from build123d import *

# Parameters (mm, degrees)
SKETCH1_W           = 38.1
SKETCH1_H           = 38.1
SKETCH1_R           = 1.0795
BOSS_EXTRUDE1_DEPTH = 1.5875
SKETCH3_W           = 10.16
SKETCH3_H           = 5.08
BOSS_EXTRUDE2_DEPTH = 8.89
SKETCH4_R           = 8.255
BOSS_EXTRUDE3_DEPTH = 16.637


with BuildPart() as part:
    # Sketch1 → Boss-Extrude1 (new body)
    with BuildSketch(Plane(origin=(0, 0, 0), x_dir=(0, 0, -1), z_dir=(1, 0, 0))):
        Rectangle(SKETCH1_W, SKETCH1_H)
        with Locations((13.97, -13.97)):
            Circle(SKETCH1_R, mode=Mode.SUBTRACT)
        with Locations((-13.97, -13.97)):
            Circle(SKETCH1_R, mode=Mode.SUBTRACT)
        with Locations((-13.97, 13.97)):
            Circle(SKETCH1_R, mode=Mode.SUBTRACT)
        with Locations((13.97, 13.97)):
            Circle(SKETCH1_R, mode=Mode.SUBTRACT)
    extrude(amount=BOSS_EXTRUDE1_DEPTH)

    # Sketch3 → Boss-Extrude2 (add)
    with BuildSketch(Plane.ZY):
        with Locations((-6.35, -12.7)):
            Rectangle(SKETCH3_W, SKETCH3_H)
    extrude(amount=BOSS_EXTRUDE2_DEPTH)

    # Sketch4 → Boss-Extrude3 (add)
    with BuildSketch(Plane(origin=(1.5875, 0, 0), x_dir=(0, 0, -1), z_dir=(1, 0, 0))):
        Circle(SKETCH4_R)
    extrude(amount=BOSS_EXTRUDE3_DEPTH)


solid = part.part
The listing builds one solid part. Answer for the finished solid, in the listing's coordinates (mm). A direction names the side the tool comes from. Coordinates: 2 decimals unless noted, no trailing zeros. Loops run counter-clockwise (first coordinate to the right, second up) from the corner with the lowest first, then second, coordinate; pieces in that order, holes last. Notation, with made-up numbers: (-19.75, 69) -> (33.25, 69) arc R18 ccw to (33.25, 94) -> close; hole circle Ø2 at (81, 71). An arc over 180 degrees is marked (long way). Answer in a Markdown table with one row per item. Add a question column.
1. For faces 1 (the flat face through (-4, -15.24, -6)), 2 (the flat face through (-4, -13, -1.27)), 3 (the flat face through (-4, -10.16, -6)), 4 (the cylindrical face through (9.79, 2.48, -7.874)), determine the directions among +Z, -Z, +X, -X, +Y, -Y from which every point of the face is accessible in a straight line to the end or side of a thin tool.
2. The part is cut by section D-D, the plane x = -5.75. Write down the section's boundary in (y, z).
3. Determine the mould class of faces 5 (the flat face through (-4, -13, -11.43)), 6 (the flat face through (1, -19.05, 0)), 7 (the cylindrical face through (0.78, -14.38, -14.97)) for opening direction Z: +Z half, -Z half, draft (parallel to the pull), parting line (faces both ways), or undercut.
4. The part is cut by section B-B, the plane z = -13.97. Write down the section's boundary in (x, y), then the cut area to 3 significant figures.
5. Consider line 1 (Y direction, x = 1, z = -13.97); line 2 (X direction, y = -12.5, z = 12); line 3 (X direction, y = 1, z = 3.5). Determine where each line is inside the solid, lowest interval first. Write a range as [from, to].
6. Flat-ended cylindrical pins translate along their axes: P1, Ø3, axis at y = 9.5, z = -3.5, coming from the -X side; P2, Ø4.5, axis at x = -5.5, z = -5, coming from the +Y side; P3, Ø2.5, axis at x = -4, z = -6, coming from the -Y side. Find the tip coordinate at first contact, or state that the pin passes through.
7. The part is cut by section A-A, the plane y = -13.97. Write down the section's boundary in (x, z).
Answer below:
| question | item | result |
|---|---|---|
| 1 | face 1 | +Z, -Z, -X, -Y |
| 1 | face 2 | +Z, -X, +Y, -Y |
| 1 | face 3 | +Z, -Z, -X, +Y |
| 1 | face 4 | +X |
| 2 | outline | (-15.24, -11.43) -> (-10.16, -11.43) -> (-10.16, -1.27) -> (-15.24, -1.27) -> close |
| 3 | face 5 | -Z half |
| 3 | face 6 | draft |
| 3 | face 7 | undercut |
| 4 | outline | (0, -19.05) -> (1.59, -19.05) -> (1.59, -15.05) -> (0, -15.05) -> close; (0, -12.89) -> (1.59, -12.89) -> (1.59, 12.89) -> (0, 12.89) -> close; (0, 15.05) -> (1.59, 15.05) -> (1.59, 19.05) -> (0, 19.05) -> close |
| 4 | area | 53.6 mm2 |
| 5 | line 1 | [-19.05, -15.05], [-12.89, 12.89], [15.05, 19.05] |
| 5 | line 2 | [0, 1.59] |
| 5 | line 3 | [0, 18.22] |
| 6 | P1 | x = 0 |
| 6 | P2 | y = -10.16 |
| 6 | P3 | y = -15.24 |
| 7 | outline | (-8.89, -11.43) -> (0, -11.43) -> (0, -12.89) -> (1.59, -12.89) -> (1.59, 12.89) -> (0, 12.89) -> (0, -1.27) -> (-8.89, -1.27) -> close; (0, -19.05) -> (1.59, -19.05) -> (1.59, -15.05) -> (0, -15.05) -> close; (0, 15.05) -> (1.59, 15.05) -> (1.59, 19.05) -> (0, 19.05) -> close |
